The listing builds one solid part. Answer for the finished solid, in the listing's coordinates (mm). Give positions to 0.01 mm unless a question says otherwise; leave off trailing zeros. Write each loop counter-clockwise with the first axis right and the second up, starting at its lowest first coordinate (ties: lowest second). Pieces come first, ordered by that corner, then holes. Notation, with made-up numbers: (18, 54.5) - (37, 54.5) arc R20 ccw to (37, 86.5) - close; hole circle Ø4 at (29, 36). An arc over 180 degrees is marked (long way). Answer as CSV lines item,"result". Start each with the question number.
(1) Each of these flat-tipped pins is pushed along its axis until it touches: pin 1 Ø7.5 at (x, z) = (0, 0) entering from -Y; pin 2 Ø2 at (x, y) = (2.5, -3.5) entering from -Z; pin 3 Ø2 at (y, z) = (-1.5, -11) entering from +X. Where does it stop, or does it pass through?
(2) For a pull along Z with two mould halves and no side action, classify faces 1 (the face through (0, 0, -5)), 2 (the face through (-2.579, -0.616, 1.978)), 3 (the face through (23.846, -2.972, -7.509)) as pulls with the +Z half, pulls with the -Z half, needs draft (parallel to the pull), parting line crosses it, or undercut.
(3) Straight lines are drawn through the part: probe 1 along Z at (x, y) = (0, -1.2); probe 2 along Z at (x, y) = (3.5, -2.1); probe 3 along X at (y, z) = (-1.2, -1.5). For each, find the intervals that lie inside material, in ascending order.
(4) Find section A-A (z = 0). Write down the section's boundary in (x, y).
(5) Find section B-B (x = 0). Write down the section's boundary in (y, z).
(6) Find section C-C (y = -3.9). Write down the section's boundary in (x, z), then the cut area to 3 significant figures.
Solid Edge part; units mm, degrees
sketch "Sketch1" plane through (0, 0, 0) normal (0, -1, 0) x (1, 0, 0)
  circle A0 centre (0, 0) radius 25
extrude "Protrusion1" add sketch "Sketch1" along normal blind 5
chamfer "Chaflán_3" distance 1 angle 45 1 edges at (-25, 0, 0)
sketch "Sketch2" plane through (0, 0, 0) normal (0, 0, 1) x (1, 0, 0)
  line L0 (3.25, -1.25) -> (7, -5)
  line L1 (3.25, -1.25) -> (3.25, 0)
  dimension "D1" = 3.25
revolve "RevolvedCutout1" cut sketch "Sketch2" angle 360 about axis through (0, 0, 0) along (0, 1, 0) material side at (5.0896, -3.1604, 0)
properties part number "1976-1100-001" material "Aluminio, 7075-T6"
Result set:
1,pin 1,"y = -1.75"
1,pin 2,"z = -24.95"
1,pin 3,"x = 22.91"
2,face 1,"needs draft"
2,face 2,"undercut"
2,face 3,"parting line crosses it"
3,probe 1,"-25 to -3.25, 3.25 to 25"
3,probe 2,"-24.75 to -2.14, 2.14 to 24.75"
3,probe 3,"-24.95 to -2.88, 2.88 to 24.95"
4,outline,"(-25, -5) - (-7, -5) - (-3.25, -1.25) - (-3.25, 0) - (-24, 0) - (-25, -1) - close; (3.25, -1.25) - (7, -5) - (25, -5) - (25, -1) - (24, 0) - (3.25, 0) - close"
5,outline,"(-5, -25) - (-1, -25) - (0, -24) - (0, -3.25) - (-1.25, -3.25) - (-5, -7) - close; (-5, 7) - (-1.25, 3.25) - (0, 3.25) - (0, 24) - (-1, 25) - (-5, 25) - close"
6,outline,"circle Ø50 at (0, 0); hole circle Ø11.8 at (0, 0)"
6,area,"1,850 mm^2"
